from build123d import *

# Parameters (mm, degrees)
F0_R     = 10
F1_DEPTH = 5
F2_R     = 0.835
F3_DEPTH = 5.001
F3_TAPER = -3
F5_DEPTH = 5


with BuildPart() as f1:
    # F0 (on Top) → F1 (new body)
    with BuildSketch(Plane.XY):
        Circle(F0_R)
    extrude(amount=F1_DEPTH)

    # F2 (on face) → F3 (cut, through all)
    with BuildSketch(Plane.XY.offset(5)):
        Circle(F2_R)
    extrude(amount=-F3_DEPTH, taper=F3_TAPER, mode=Mode.SUBTRACT)

    # F4 (on face) → F5 (join)
    with BuildSketch(Plane(origin=(0, 0, 0), x_dir=(1, 0, 0), z_dir=(0, 0, -1))):
        Polygon((0, 20), (-3.2380346414, 7.0478614342), (-14.1421356237, 14.1421356237), (-7.0869063945, 3.2282734014), (-20, 0), (-7.0869063945, -3.2282734014), (-14.1421356237, -14.1421356237), (-3.2282734014, -7.0869063945), (0, -20), (3.2338841378, -7.0644634487), (14.21151183, -14.0724174009), (7.1094684771, -3.2226328807), (20, 0), (7.1094684771, 3.2226328807), (14.21151183, 14.0724174009), (3.2436714877, 7.0253140492), align=None)
    extrude(amount=-F5_DEPTH)


solid = f1.part
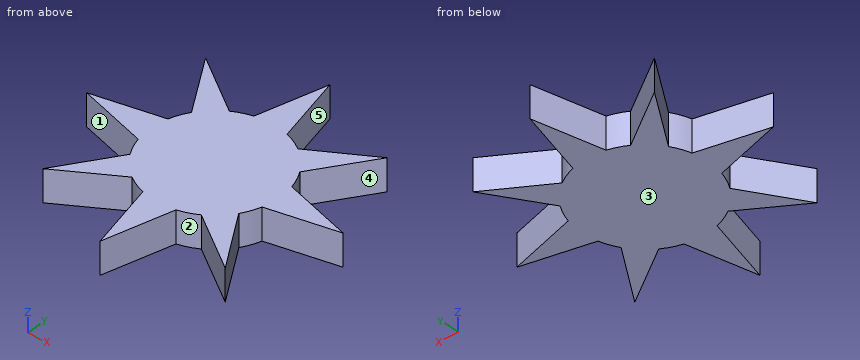
Could you check a few things on this model? Use its own coordinates, in mm. Face numbers are marked on the shaded views. A direction names the side the tool comes from. Give positions to 0.01 mm unless a question says otherwise; leave off trailing zeros. Order: outer loops, then holes, each group sorted by start corner. A loop starts at its lowest first (then second) coordinate and runs counter-clockwise, first axis right, second up. Notation, with made-up numbers: (-35, -37) - (6, -37) arc R20 ccw to (6, -30) - close; hole circle Ø10 at (32, -22.5). An arc over 180 degrees is marked (long way). Return JSON: item names as keys, results as strings. Group by question number.
Q1. Please list where these lines run through material, in increasing order: line 1 along Y through (x, z) = (13, 3.45); line 2 along Y through (x, z) = (-13, 2.7); line 3 along X through (y, z) = (12, 4.1). Write a range as [from, to].
Q2. Suppose I cut it at D-D, the plane x = 2. Please give me the cut outline in (y, z).
Q3. Will these pins go through, and if not, where does the flat tip stop? pin 1 Ø12 at (x, y) = (13, 4) entering from -Z; pin 2 Ø2 at (y, z) = (11, 1.5) entering from +X; pin 3 Ø2 at (x, z) = (-5, 1.5) entering from +Y.
Q4. Suppose I cut it at B-B, the plane z = 4.5. Please give me the cut outline in (x, y).
Q5. Suppose I cut it at A-A, the plane x = 13.5. Please give me the cut outline in (y, z) (3 decimals), and give its area (3 significant figures).
Q6. Suppose I cut it at C-C, the plane y = 1.5. Please give me the cut outline in (x, z).
Q7. Which directions (+Z, -Z, +X, -X, +Y, -Y) give clear straight access to the entire face, cutting with the end or side of a thin tool? Please do the marked faces 1, 2, 3, 4 and 5.
Resolved:
{
 "1": {"line 1": "y = [-13.29, -12.22], [-1.75, 1.75], [12.22, 13.3]", "line 2": "y = [-13.4, -12.38], [-1.75, 1.75], [12.38, 13.4]", "line 3": "x = [-12.76, -10.83], [-2, 2], [10.97, 12.85]"},
 "2": {"outline": "(-12, 0) - (12, 0) - (12, 5) - (-12, 5) - close"},
 "3": {"pin 1": "stops at z = 0", "pin 2": "stops at x = 12.85", "pin 3": "stops at y = 9.17"},
 "4": {"outline": "(-20, 0) - (-9.66, -2.58) arc R10 ccw to (-8.45, -5.34) - (-14.14, -14.14) - (-5.37, -8.44) arc R10 ccw to (-2.58, -9.66) - (0, -20) - (2.58, -9.66) arc R10 ccw to (5.4, -8.41) - (14.21, -14.07) - (8.47, -5.31) arc R10 ccw to (9.66, -2.58) - (20, 0) - (9.66, 2.58) arc R10 ccw to (8.47, 5.31) - (14.21, 14.07) - (5.38, 8.43) arc R10 ccw to (2.58, 9.66) - (0, 20) - (-2.58, 9.66) arc R10 ccw to (-5.34, 8.45) - (-14.14, 14.14) - (-8.45, 5.34) arc R10 ccw to (-9.66, 2.58) - close"},
 "5": {"outline": "(-13.615, 0) - (-12.985, 0) - (-12.985, 5) - (-13.615, 5) - close; (-1.625, 0) - (1.625, 0) - (1.625, 5) - (-1.625, 5) - close; (12.985, 0) - (13.618, 0) - (13.618, 5) - (12.985, 5) - close", "area": "22.6 mm2"},
 "6": {"outline": "(-14, 0) - (14, 0) - (14, 5) - (-14, 5) - close"},
 "7": {"face 1": "+Z, -Z, -X", "face 2": "+Z, -Z, -Y", "face 3": "-Z, +X, -X, +Y, -Y", "face 4": "+Z, -Z, +X", "face 5": "+Z, -Z, +Y"}
}
